The listing builds one solid part. Answer for the finished solid, in the listing's coordinates (mm). A direction names the side the tool comes from. Coordinates: 2 decimals unless noted, no trailing zeros. Order: outer loops, then holes, each group sorted by start corner. A loop starts at its lowest first (then second) coordinate and runs counter-clockwise, first axis right, second up. Notation, with made-up numbers: (71.25, -34.5) - (124.25, -34.5) arc R20 cw to (124.25, -1.5) - close; hole circle Ø5 at (21, -24.75). An arc over 180 degrees is marked (long way). Use a Markdown table: item, result. Add a question column.
Item 1: Find the intervals of material crossed by line 1 along Z through (x, y) = (18.5, 10.75); line 2 along Z through (x, y) = (-4, 15); line 3 along X through (y, z) = (8.5, 5) (3 decimals), in increasing order.
Item 2: The part is cut by section B-B, the plane y = 20.5. Give the vertices of the cut face in (x, z), then the cut area to 3 significant figures.
Item 3: For faces 1 (the flat face through (15.3, 9.8, 6.223)), 2 (the flat face through (20, 5.916, 12)), 3 (the flat face through (1, 12.266, 8)), 4 (the flat face through (20, 8, 5.08)), 5 (the flat face through (5, 14.806, 3)), determine the directions among +Z, -Z, +X, -X, +Y, -Y from which every point of the face is accessible in a straight line to the end or side of a thin tool.
Item 4: The part is cut by section C-C, the plane x = 4.5. Give the vertices of the cut face in (y, z), then the cut area to 3 significant figures.
Item 5: The part is cut by section D-D, the plane x = -6.5. Give the vertices of the cut face in (y, z).
Item 6: Flat-ended cylindrical pins translate along their axes: P1, Ø1.6, axis at x = 0, z = 14, coming from the +Y side; P2, Ø2, axis at y = 18, z = 14, coming from the -X side; P3, Ø1.5, axis at x = 1, y = 21.5, coming from the +Z side; P4, Ø0.6, axis at x = 20.5, y = 8.5, coming from the -Z side. Find the tip coordinate at first contact, or state that the pin passes through.
Item 7: The mould has two halves that part along X. Classify faces 6 (the flat face through (16.06, 19.85, 8.15)), 7 (the cylindrical face through (17.98, 11.25, 11.37)), 8 (the flat face through (20, 5.916, 4)): released by +X, released by -X, zero draft, split by the parting line, or undercut.
from build123d import *

# Parameters (mm, degrees)
F1_DEPTH  = 16.383
F2_W      = 33.528
F2_H      = 5.969
F3_DEPTH  = 11.43
F4_SIZE   = 11.43
F5_R      = 2.159
F6_DEPTH  = 25.4
F8_DEPTH  = 6.35
F10_DEPTH = 10.16
F11_R     = 6.34999
F12_W     = 4.191
F12_H     = 2.54
F12_H_2   = 1.905
F13_DEPTH = 2.667
F14_R     = 5.08


# Not quite as in the source:
# - a fillet or chamfer is up to 0.001 mm smaller than in the source, because OpenCascade refuses the exact size


with BuildPart() as f1:
    # F0 (on Top) → F1 (new body)
    with BuildSketch(Plane.XY):
        Polygon((21.1023603916, 14.8059087365), (-12.4256396084, 14.8059087365), (-12.4256396084, 5.9159087365), (-9.8856396084, 5.9159087365), (-9.8856396084, 12.2659087365), (11.7043603916, 12.2659087365), (11.7043603916, 5.9159087365), (21.1023603916, 5.9159087365), align=None)
    extrude(amount=F1_DEPTH)

    # F2 (on face) → F3 (join)
    with BuildSketch(Plane(origin=(0, 14.8059087365, 0), x_dir=(-1, 0, 0), z_dir=(0, 1, 0))):
        with Locations((-4.3383603916, 8.1915)):
            Rectangle(F2_W, F2_H)
    extrude(amount=F3_DEPTH)

    # F4
    f4_edges = [f1.edges().sort_by_distance(p)[0] for p in [
        (-12.42564, 26.235909, 8.1915),
        (21.10236, 26.235909, 8.1915),
    ]]
    chamfer(f4_edges, length=F4_SIZE)

    # F5 (on face) → F6 (cut)
    with BuildSketch(Plane(origin=(0, 0, 5.207), x_dir=(1, 0, 0), z_dir=(0, 0, -1))):
        with Locations((4.3383603916, -19.8859087365)):
            Circle(F5_R)
    extrude(amount=-F6_DEPTH, mode=Mode.SUBTRACT)

    # F7 (on face) → F8 (cut)
    with BuildSketch(Plane(origin=(0, 0, 0), x_dir=(1, 0, 0), z_dir=(0, 0, -1))):
        with BuildLine():
            Line((18.5677868823, -9.6751087365), (19.2306352681, -5.9159087365))
            Line((19.2306352681, -5.9159087365), (14.846085515, -5.9159087365))
            Line((14.846085515, -5.9159087365), (15.5089339009, -9.6751087365))
            Line((15.5089339009, -9.6751087365), (15.5218644869, -9.6751087365))
            ThreePointArc((15.5218644869, -9.6751087365), (16.101190374, -10.4723310604), (17.0383603916, -10.1675454388))
            ThreePointArc((17.0383603916, -10.1675454388), (17.9755304092, -10.4723310604), (18.5548562962, -9.6751087365))
            Line((18.5548562962, -9.6751087365), (18.5677868823, -9.6751087365))
        make_face()
    extrude(amount=-F8_DEPTH, mode=Mode.SUBTRACT)

    # F9 (on face) → F10 (cut)
    with BuildSketch(Plane.XY.offset(16.383)):
        with BuildLine():
            Line((14.3731213639, 5.9159087365), (19.7035994193, 5.9159087365))
            Line((19.7035994193, 5.9159087365), (18.9287834006, 10.3101087365))
            Line((18.9287834006, 10.3101087365), (18.9070608822, 10.4264149788))
            ThreePointArc((18.9070608822, 10.4264149788), (17.9577526403, 11.2497597634), (17.0383603916, 10.3931381052))
            ThreePointArc((17.0383603916, 10.3931381052), (16.1426669703, 11.2490386173), (15.1767129861, 10.4733032939))
            Line((15.1767129861, 10.4733032939), (15.1479373825, 10.3101087365))
            Line((15.1479373825, 10.3101087365), (14.3731213639, 5.9159087365))
        make_face()
    extrude(amount=-F10_DEPTH, mode=Mode.SUBTRACT)

    # F11 (radius 6.35 in the source; OpenCascade refuses exactly that, so slightly less here)
    f11_edges = [f1.edges().sort_by_distance(p)[0] for p in [
        (11.70436, 12.265909, 8.1915),
        (-9.88564, 12.265909, 8.1915),
    ]]
    fillet(f11_edges, radius=F11_R)

    # F12 (on face) → F13 (cut)
    with BuildSketch(Plane.YZ.offset(21.1023603916)):
        with Locations((8.0114087365, 1.27)):
            Rectangle(F12_W, F12_H)
        with Locations((8.0114087365, 6.0325)):
            Rectangle(F12_W, F12_H_2)
    extrude(amount=-F13_DEPTH, mode=Mode.SUBTRACT)

    # F14
    f14_edges = [f1.edges().sort_by_distance(p)[0] for p in [
        (9.67236, 26.235909, 8.1915),
        (-0.99564, 26.235909, 8.1915),
    ]]
    fillet(f14_edges, radius=F14_R)


solid = f1.part
Solution:
| question | item | result |
|---|---|---|
| 1 | line 1 | z = 0 to 6.22 |
| 1 | line 2 | z = 5.21 to 11.18 |
| 1 | line 3 | x = -12.426 to -9.336, 11.155 to 15.302, 18.775 to 21.102 |
| 2 | outline | (-6.73, 5.21) - (2.27, 5.21) - (2.27, 11.18) - (-6.73, 11.18) - close; (6.41, 5.21) - (15.41, 5.21) - (15.41, 11.18) - (6.41, 11.18) - close |
| 2 | area | 107 mm2 |
| 3 | face 1 | +Z, -Y |
| 3 | face 2 | +Z, -Z, +X, -X, -Y |
| 3 | face 3 | +Z, -Z, -Y |
| 3 | face 4 | +X, -Y |
| 3 | face 5 | -Z, +X, -X, +Y |
| 4 | outline | (12.27, 0) - (14.81, 0) - (14.81, 5.21) - (17.73, 5.21) - (17.73, 11.18) - (14.81, 11.18) - (14.81, 16.38) - (12.27, 16.38) - close; (22.04, 5.21) - (26.24, 5.21) - (26.24, 11.18) - (22.04, 11.18) - close |
| 4 | area | 84.1 mm2 |
| 5 | outline | (11.53, 0) - (14.81, 0) - (14.81, 5.21) - (20.73, 5.21) - (20.73, 11.18) - (14.81, 11.18) - (14.81, 16.38) - (11.53, 16.38) - close |
| 6 | P1 | stops at y = 14.81 |
| 6 | P2 | passes through |
| 6 | P3 | stops at z = 11.18 |
| 6 | P4 | stops at z = 2.54 |
| 7 | face 6 | released by +X |
| 7 | face 7 | undercut |
| 7 | face 8 | zero draft |
